The figure shows three views and two pictorial views of one solid part (mm, origin at its lowest corner). Answer the questions. Round coordinates to 2 decimals unless told otherwise and drop trailing zeros. Order: outer loops, then holes, each group sorted by start corner. A loop starts at its lowest first (then second) coordinate and runs counter-clockwise, first axis right, second up. Notation, with made-up numbers: (85.5, -27) -> (94.5, -27) arc R6 ccw to (94.5, -21) -> close; hole circle Ø1 at (10, 31). An arc over 180 degrees is marked (long way). Answer as a JSON object with one key per item and string values. Group by question number.
Item 1: Consider probe 1 along X at (y, z) = (0.6, 12.5) (3 decimals); probe 2 along Z at (x, y) = (10, 0.7) (1 decimal); probe 3 along X at (y, z) = (0.95, 21.75). Determine where each line is inside the solid, lowest interval first. Write a range as from..to.
Item 2: Section C-C, the plane z = 17.25 is taken. Write down the section's boundary in (x, y).
Item 3: Section A-A, the plane x = 12.5 is taken. Write down the section's boundary in (y, z) (3 decimals).
Item 4: Section B-B, the plane y = 0.6 is taken. Count the separate pieces of the cut face and the enclosed holes in it.
Item 5: Section D-D, the plane z = 21.5 is taken. Write down the section's boundary in (x, y) (1 decimal).
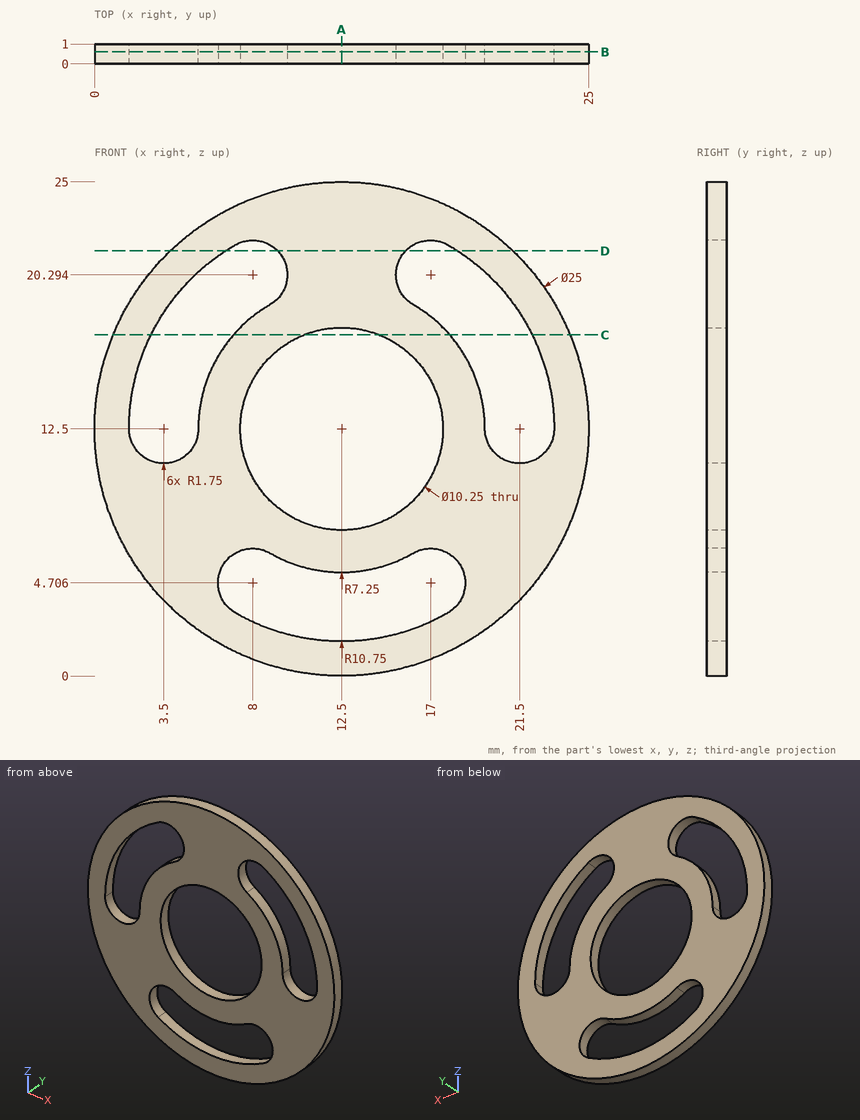
Values found:
{
 "1": {"probe 1": "0..1.75, 5.25..7.375, 17.625..19.75, 23.25..25", "probe 2": "0.3..2, 5.7..8, 17..24.7", "probe 3": "4.09..7.02, 8.97..16.03, 17.98..20.91"},
 "2": {"outline": "(0.94, 0) -> (2.86, 0) -> (2.86, 1) -> (0.94, 1) -> close; (7.02, 0) -> (10.58, 0) -> (10.58, 1) -> (7.02, 1) -> close; (14.42, 0) -> (17.98, 0) -> (17.98, 1) -> (14.42, 1) -> close; (22.14, 0) -> (24.06, 0) -> (24.06, 1) -> (22.14, 1) -> close"},
 "3": {"outline": "(0, 0) -> (1, 0) -> (1, 1.75) -> (0, 1.75) -> close; (0, 5.25) -> (1, 5.25) -> (1, 7.375) -> (0, 7.375) -> close; (0, 17.625) -> (1, 17.625) -> (1, 25) -> (0, 25) -> close"},
 "4": {"separate pieces": "1", "enclosed holes": "4"},
 "5": {"outline": "(3.8, 0) -> (6.6, 0) -> (6.6, 1) -> (3.8, 1) -> close; (9.3, 0) -> (15.7, 0) -> (15.7, 1) -> (9.3, 1) -> close; (18.4, 0) -> (21.2, 0) -> (21.2, 1) -> (18.4, 1) -> close"}
}
